Input: part model. Units: mm. Frame: model coordinates. A direction names the side the tool comes from. Round coordinates to 2 decimals unless told otherwise and drop trailing zeros. Loops run counter-clockwise (first coordinate to the right, second up) from the corner with the lowest first, then second, coordinate; pieces in that order, holes last.
1) Draft query along Y for faces 1 (the face through (-2.44, -0.54, -27.88)), 2 (the face through (1.983, 0, 3)), 3 (the face through (-2, 2, 5.1)). Return one class per face: pulls with the +Y half, pulls with the -Y half, needs draft (parallel to the pull), parting line crosses it, or undercut.
2) Access query for faces 4 (the face through (-2, 2, 0)), 5 (the face through (0.978, 1.726, 3.128)), 6 (the face through (0, 0, -55)). Directions: +Z, -Z, +X, -X, +Y, -Y. A direction counts if a zero-diameter tool reaches every point of the face in a straight line with its end or side. Return the directions, or none.
3) Section B-B, the plane z = -5.5. Return loops of the section in (x, y), and give its area (3 significant figures).
4) Section A-A, the plane y = 0. Return loops of the section in (x, z), and give its area (3 significant figures).
5) First-contact query: pin 1 (4.5 mm diameter, centred on x = 0.5, y = 0.5, fed in from +Z); pin 2 (1.5 mm diameter, centred on y = 3.5, z = -48.5, fed in from -X); pin 3 (1 mm diameter, centred on y = -2, z = -36.5, fed in from -X); pin 4 (2 mm diameter, centred on y = 1, z = -18.5, fed in from +X). Flat tips, straight axial feed; report the tip coordinate or a pass-through.
6) Ray query, line 1 along Z through (x, y) = (-1.5, -1); line 2 along Z through (x, y) = (1.5, -2.5); line 3 along Y through (x, z) = (-1, -16). Return the intervals inside material, ascending.
Autodesk Inventor part; units mm, degrees
ref_plane "YZ Plane" through (0, 0, 0) normal (1, 0, 0) x (0, 1, 0)
ref_plane "XZ Plane" through (0, 0, 0) normal (0, 1, 0) x (-1, 0, 0)
ref_plane "XY Plane" through (0, 0, 0) normal (0, 0, 1) x (1, 0, 0)
sketch "スケッチ1" plane through (0, 0, 0) normal (1, 0, 0) x (0, 1, 0)
  line L0 (4.3, 5.1) -> (4.3, 0)
  line L1 (4.3, 0) -> (2.5, 0)
  line L2 (2.5, 0) -> (2.5, -55)
  line L3 (0, -55) -> (2.5, -55)
  line L4 (4.3, 5.1) -> (0, 5.1)
  line L5 (0, 5.1) -> (0, -55)
  point P0 (0, 0)
  dimension "d2" = 0
  dimension "d3" = 55
  dimension "d4" = 4.3
  dimension "d5" = 5.1
  dimension "d6" = 0
  dimension "d7" = 2.5
revolve "回転1" add sketch "スケッチ1" angle 360 about axis through (0, 0, 5.1) along (0, 0, -1)
chamfer "面取り1" distance 0.5 angle 45 1 edges at (0, -4.3, 5.1)
sketch "スケッチ2" plane through (0, 0, 5.1) normal (0, 0, 1) x (1, 0, 0)
  circle A0 centre (0, 0) radius 2.29
  line L0 (0, 0) -> (-2.9175, 1.6844)
  line L1 (0, 0) -> (-1.7508, 0)
  point P0 (0, 0)
  point P1 (-1.9832, 1.145)
  point P2 (-1.9832, -1.145)
  point P3 (0, -2.29)
  point P4 (1.9832, -1.145)
  point P5 (1.9832, 1.145)
  point P6 (0, 2.29)
  dimension "d12" = 4.58
  dimension "d14" = 30
  dimension "d21" = 360
sketch "スケッチ3" plane through (0, 0, 5.1) normal (0, 0, 1) x (1, 0, 0)
  line L0 (-1.9832, 1.145) -> (0, 2.29)
  line L1 (0, 2.29) -> (1.9832, 1.145)
  line L2 (1.9832, 1.145) -> (1.9832, -1.145)
  line L3 (1.9832, -1.145) -> (0, -2.29)
  line L4 (0, -2.29) -> (-1.9832, -1.145)
  line L5 (-1.9832, -1.145) -> (-1.9832, 1.145)
  point P0 (0, 0)
  point P1 (-2.5, -1.3891)
extrude "押し出し1" cut sketch "スケッチ3" against normal blind 4
thread "ねじ1"
sketch "スケッチ4" plane through (0, 0, 0) normal (0, 1, 0) x (-1, 0, 0)
  line L0 (-3.8, 5.1) -> (3.8, 5.1)
  line L1 (0, 5.1) -> (0, 1.1)
  line L2 (2.29, 5.1) -> (1.9832, 4.7932)
  line L3 (1.9832, 5.1) -> (1.9832, 1.1)
  line L4 (1.9832, 5.1) -> (2.29, 5.1)
  point P0 (0, 0)
  dimension "d27" = 2.29
  dimension "d28" = 45
revolve "回転2" cut sketch "スケッチ4" angle 360 about axis through (0, 0, 5.1) along (0, 0, -1)
properties part number "CB5-55" material "鋼、炭素鋼"
Final values:
1. face 1: parting line crosses it
1. face 2: undercut
1. face 3: needs draft
2. face 4: -Z
2. face 5: +Z
2. face 6: -Z, +X, -X, +Y, -Y
3. outline: circle Ø5 at (0, 0)
3. area: 19.6 mm2
4. outline: (-4.3, 0) - (-2.5, 0) - (-2.5, -55) - (2.5, -55) - (2.5, 0) - (4.3, 0) - (4.3, 4.6) - (3.8, 5.1) - (2.29, 5.1) - (1.98, 4.79) - (1.98, 1.1) - (-1.98, 1.1) - (-1.98, 4.79) - (-2.29, 5.1) - (-3.8, 5.1) - (-4.3, 4.6) - close
4. area: 303 mm2
5. pin 1: stops at z = 5.1
5. pin 2: passes through
5. pin 3: stops at x = -2
5. pin 4: stops at x = 2.5
6. line 1: z = -55 to 1.1
6. line 2: z = 0 to 5.1
6. line 3: y = -2.29 to 2.29
